from build123d import *

# Parameters (mm, degrees)
SKETCH1_W                        = 203.2
SKETCH1_H                        = 25.4
BOSS_EXTRUDE1_DEPTH              = 6.35
F_5_8_0_625_DIAMETER_HOLE1_D     = 15.875
F_5_8_0_625_DIAMETER_HOLE1_DEPTH = 25.4
F_5_8_0_625_DIAMETER_HOLE1_TIP   = 4.769331164
CUT_EXTRUDE1_DEPTH               = 7.35
CUT_EXTRUDE2_DEPTH               = 3.175
F_4_CLEARANCE_HOLE1_D            = 3.2639


with BuildPart() as part:
    # Sketch1 → Boss-Extrude1 (new body)
    with BuildSketch(Plane(origin=(0, 0, 0), x_dir=(1, 0, 0), z_dir=(0, 1, 0))):
        with Locations((101.6, 12.7)):
            Rectangle(SKETCH1_W, SKETCH1_H)
    extrude(amount=BOSS_EXTRUDE1_DEPTH)

    # 5/8 (0.625) Diameter Hole1
    with Locations(Plane(origin=(0, 6.35, 0), x_dir=(1, 0, 0), z_dir=(0, 1, 0))):
        with Locations((101.6, 12.7)):
            Hole(F_5_8_0_625_DIAMETER_HOLE1_D / 2, depth=F_5_8_0_625_DIAMETER_HOLE1_DEPTH)
            with Locations((0, 0, -(F_5_8_0_625_DIAMETER_HOLE1_DEPTH + F_5_8_0_625_DIAMETER_HOLE1_TIP / 2))):  # 118° drill point
                Cone(0, F_5_8_0_625_DIAMETER_HOLE1_D / 2, F_5_8_0_625_DIAMETER_HOLE1_TIP, mode=Mode.SUBTRACT)

    # Sketch6 → Cut-Extrude1 (cut, through all)
    with BuildSketch(Plane(origin=(0, 6.35, 0), x_dir=(1, 0, 0), z_dir=(0, 1, 0))):
        with BuildLine():
            Line((133.35, 16.3576), (190.5, 16.3576))
            ThreePointArc((190.5, 16.3576), (194.1576, 12.7), (190.5, 9.0424))
            Line((190.5, 9.0424), (133.35, 9.0424))
            ThreePointArc((133.35, 9.0424), (129.6924, 12.7), (133.35, 16.3576))
        make_face()
    extrude(amount=-CUT_EXTRUDE1_DEPTH, mode=Mode.SUBTRACT)

    # Sketch7 → Cut-Extrude2 (cut)
    with BuildSketch(Plane(origin=(0, 6.35, 0), x_dir=(1, 0, 0), z_dir=(0, 1, 0))):
        with BuildLine():
            Line((190.5, 6.35), (133.35, 6.35))
            ThreePointArc((133.35, 6.35), (127, 12.7), (133.35, 19.05))
            Line((133.35, 19.05), (190.5, 19.05))
            ThreePointArc((190.5, 19.05), (196.85, 12.7), (190.5, 6.35))
        make_face()
    extrude(amount=-CUT_EXTRUDE2_DEPTH, mode=Mode.SUBTRACT)

    # #4 Clearance Hole1 (through all)
    with Locations(Plane(origin=(0, 6.35, 0), x_dir=(1, 0, 0), z_dir=(0, 1, 0))):
        with Locations((2.54, 22.86), (22.86, 22.86), (22.86, 2.54), (2.54, 2.54)):
            Hole(F_4_CLEARANCE_HOLE1_D / 2)


solid = part.part
Input: part model. Units: mm. Frame: model coordinates. A direction names the side the tool comes from. Coordinates: 2 decimals unless noted, no trailing zeros. Order: outer loops, then holes, each group sorted by start corner. A loop starts at its lowest first (then second) coordinate and runs counter-clockwise, first axis right, second up. Notation, with made-up numbers: M 27,8.5 L 35,8.5 A9 cw 35,15.5 Z; hole C 6.5,53 d4. An arc over 180 degrees is marked long. Answer in a Markdown table with one row per item.
(1) Access query for faces 1 (the flat face through (100, 0, -21)), 2 (the cylindrical face through (127, 4.8, -12.6)), 3 (the flat face through (162, 2, -9.042)). Directions: +Z, -Z, +X, -X, +Y, -Y. A direction counts if a zero-diameter tool reaches every point of the face in a straight line with its end or side. Return the directions, or none.
Numbers:
| item | result |
|---|---|
| face 1 | +Z, -Z, +X, -X, -Y |
| face 2 | +Y |
| face 3 | +Y, -Y |
(2) Draft query along X for faces 4 (the flat face through (0, 3, -13)), 5 (the cylindrical face through (194.157, 1.61, -12.78)), 6 (the flat face through (100, 3, -25.4)), 7 (the flat face through (203.2, 3, -13)). Return one class per face: pulls with the +X half, pulls with the -X half, needs draft (parallel to the pull), parting line crosses it, or undercut.
Numbers:
| item | result |
|---|---|
| face 4 | pulls with the -X half |
| face 5 | undercut |
| face 6 | needs draft |
| face 7 | pulls with the +X half |
(3) Material intervals for line 1 (Z direction, x = 2.54, y = 3.5); line 2 (X direction, y = 4, z = -22.86); line 3 (Z direction, x = 149.5, y = 5), sorted ascending. Write a range as [from, to].
Numbers:
| item | result |
|---|---|
| line 1 | z = [-25.4, -24.49], [-21.23, -4.17], [-0.91, 0] |
| line 2 | x = [0, 0.91], [4.17, 21.23], [24.49, 203.2] |
| line 3 | z = [-25.4, -19.05], [-6.35, 0] |
(4) Section query A-A, the plane z = -12.7. Give the number of separate pieces and of enclosed holes in the cut face, plus the area to 3 significant figures.
Numbers:
| item | result |
|---|---|
| separate pieces | 3 |
| enclosed holes | 0 |
| area | 763 mm^2 |
(5) Section query C-C, the plane x = 98.5. Output: boundary loops of the cut face in (y, z), plus the area to 3 significant figures.
Numbers:
| item | result |
|---|---|
| outline | M 0,-25.4 L 6.35,-25.4 L 6.35,-20.01 L 0,-20.01 Z; M 0,-5.39 L 6.35,-5.39 L 6.35,0 L 0,0 Z |
| area | 68.5 mm^2 |
(6) Contact query for a flat-ended pin moving along its axis: pin 1 Ø10 at (x, z) = (154.5, -13) entering from +Y (3 decimals). Output: stop coordinate, or through.
Numbers:
| item | result |
|---|---|
| pin 1 | stops at y = 3.175 |
